Design review of the part built by this model. Coordinates are the model's own, in mm. A direction names the side the tool comes from. Round coordinates to 2 decimals unless told otherwise and drop trailing zeros. Order: outer loops, then holes, each group sorted by start corner. A loop starts at its lowest first (then second) coordinate and runs counter-clockwise, first axis right, second up. Notation, with made-up numbers: M -6.75,25.5 L 25.25,25.5 A10 ccw 25.25,39.5 Z; hole C -1,-33.75 d8. An arc over 180 degrees is marked long. Use a Markdown table: item, result. Add a question column.
(1) The part is to be moulded in two halves that separate along Y. For faces 4 (the face through (0, 6.8, -7)), 5 (the face through (7.6, -10, -7)), 6 (the face through (6.079, 4.995, -6.986)), 7 (the face through (-9, -6.8, -7)), say which applies: released by +Y, released by -Y, zero draft, split by the parting line, or undercut.
(2) Take a section at A-A (x = 7). Write out the cut boundary in (y, z).
(3) To check wall thickness, follow probe 1 along Y at (x, z) = (-7, -7.45); probe 2 along X at (y, z) = (4, -7.15); probe 3 along X at (y, z) = (-7, -6.9). State the ranges of each line that lie inside material, in increasing order. Write a range as from..to.
(4) Take a section at B-B (y = 4.15). Write out the cut boundary in (x, z).
(5) Take a section at C-C (z = -7.6). Write out the cut boundary in (x, y).
(6) For pin 1 (1 mm diameter, centred on x = -8.5, z = -7, fed in from -Y), flat-tipped, find the tip position at first contact; note if it passes through.
(7) Take a section at D-D (y = -9.75). Write out the cut boundary in (x, z), then the cut area to 3 significant figures.
(8) Machinability: for faces 1 (the face through (9, -6.8, -7)), 2 (the face through (-7.921, 4.995, -6.986)), 3 (the face through (-7.6, -10, -7)), which of the approach directions +Z, -Z, +X, -X, +Y, -Y give a long, thin tool a straight path to every point of the face, cutting with its end or side? Answer none if there is none.
```python
from build123d import *

# Parameters (mm, degrees)
SKETCH003_W     = 19.3
SKETCH003_H     = 13.6
PAD002_DEPTH    = 2
SKETCH004_W     = 15.2
SKETCH004_H     = 5.5
PAD003_DEPTH    = 2
SKETCH005_R     = 1.25
POCKET001_DEPTH = 5


with BuildPart() as part:
    # Sketch003 → Pad002 (new body)
    with BuildSketch(Plane.XY):
        Rectangle(SKETCH003_W, SKETCH003_H)
    extrude(amount=PAD002_DEPTH)

    # Sketch004 (on Face6 of Pad002) → Pad003 (join)
    with BuildSketch(Plane.XY.offset(2)):
        with Locations((0, -9.55)):
            Rectangle(SKETCH004_W, SKETCH004_H)
    extrude(amount=-PAD003_DEPTH)

    # Sketch005 (on Face5 of Pad003) → Pocket001 (cut)
    with BuildSketch(Plane.XY.offset(2)):
        with Locations((-7, 4.15)):
            Circle(SKETCH005_R)
        with Locations((7, 4.15)):
            Circle(SKETCH005_R)
    extrude(amount=-POCKET001_DEPTH, mode=Mode.SUBTRACT)


with BuildPart() as part_1:
    # Body001 placement: moved
    add(part.part.moved(Location((0, 0, -8))))


solid = part_1.part
```
Verdict:
| question | item | result |
|---|---|---|
| 1 | face 4 | released by +Y |
| 1 | face 5 | zero draft |
| 1 | face 6 | undercut |
| 1 | face 7 | released by -Y |
| 2 | outline | M -12.3,-8 L 2.9,-8 L 2.9,-6 L -12.3,-6 Z; M 5.4,-8 L 6.8,-8 L 6.8,-6 L 5.4,-6 Z |
| 3 | probe 1 | y = -12.3..2.9, 5.4..6.8 |
| 3 | probe 2 | x = -9.65..-8.24, -5.76..5.76, 8.24..9.65 |
| 3 | probe 3 | x = -7.6..7.6 |
| 4 | outline | M -9.65,-8 L -8.25,-8 L -8.25,-6 L -9.65,-6 Z; M -5.75,-8 L 5.75,-8 L 5.75,-6 L -5.75,-6 Z; M 8.25,-8 L 9.65,-8 L 9.65,-6 L 8.25,-6 Z |
| 5 | outline | M -9.65,-6.8 L -7.6,-6.8 L -7.6,-12.3 L 7.6,-12.3 L 7.6,-6.8 L 9.65,-6.8 L 9.65,6.8 L -9.65,6.8 Z; hole C -7,4.15 d2.5; hole C 7,4.15 d2.5 |
| 6 | pin 1 | stops at y = -6.8 |
| 7 | outline | M -7.6,-8 L 7.6,-8 L 7.6,-6 L -7.6,-6 Z |
| 7 | area | 30.4 mm^2 |
| 8 | face 1 | +Z, -Z, +X, -Y |
| 8 | face 2 | +Z, -Z |
| 8 | face 3 | +Z, -Z, -X, -Y |
